from build123d import *

# Parameters (mm, degrees)
PAD_DEPTH     = 26.9875
SKETCH001_R   = 25
SKETCH001_R_2 = 15.925
PAD001_DEPTH  = 35
SKETCH002_R   = 25
SKETCH002_R_2 = 20
PAD002_DEPTH  = 381
SKETCH003_R   = 3.175
POCKET_DEPTH  = 12.7


with BuildPart() as part:
    # Sketch → Pad (new body, symmetric)
    with BuildSketch(Plane.YZ):
        Polygon((-25.4, -76.2), (-139.7, -76.2), (-139.7, 0), (0, 0), (0, -50.8), align=None)
    extrude(amount=PAD_DEPTH, both=True)

    # Sketch001 (on Face3 of Pad) → Pad001 (join)
    with BuildSketch(Plane(origin=(0, 0, 0), x_dir=(0, -1, 0), z_dir=(0, 0, 1))):
        with Locations((65, 0)):
            Circle(SKETCH001_R)
        with Locations((65, 0)):
            Circle(SKETCH001_R_2, mode=Mode.SUBTRACT)
    extrude(amount=PAD001_DEPTH)

    # Sketch002 → Pad002 (join)
    with BuildSketch(Plane.XZ):
        with Locations((0, -35.194401)):
            Circle(SKETCH002_R)
        with Locations((0, -35.194401)):
            Circle(SKETCH002_R_2, mode=Mode.SUBTRACT)
    extrude(amount=PAD002_DEPTH)

    # Sketch003 (on Face1 of Pad002) → Pocket (cut)
    with BuildSketch(Plane.YX.offset(76.2)):
        with Locations((-127, 0)):
            Circle(SKETCH003_R)
        with Locations((-95.25, 0)):
            Circle(SKETCH003_R)
    extrude(amount=-POCKET_DEPTH, mode=Mode.SUBTRACT)


solid = part.part
Verification items for the finished model (mm, model axes). A direction names the side the tool comes from. Coordinates: 2 decimals unless noted, no trailing zeros. Order: outer loops, then holes, each group sorted by start corner. A loop starts at its lowest first (then second) coordinate and runs counter-clockwise, first axis right, second up. Notation, with made-up numbers: M -33.75,8 L -7.75,8 A22 ccw -7.75,38 Z; hole C 72,35.25 d7. An arc over 180 degrees is marked long. Return JSON: item names as keys, results as strings.
1) Cross-section at D-D, the plane y = -150. Record the boundary of the cut face in (x, z), and give its area (3 significant figures).
Answer list:
{"outline": "C 0,-35.19 d50; hole C 0,-35.19 d40", "area": "707 mm2"}
2) Release check for a two-part mould opening along X. For faces 1 (the flat face through (0, -139.7, -64)), 2 (the cylindrical face through (-0.314, -4.159, -60.192)), 3 (the flat face through (0, -127, -63.5)) record: +X half, -X half, draft (parallel to the pull), parting line (faces both ways), or undercut.
Answer list:
{"face 1": "draft", "face 2": "parting line", "face 3": "undercut"}
3) Cross-section at B-B, the plane z = 9.5. Record the boundary of the cut face in (x, y) (3 decimals), and give its area (3 significant figures).
Answer list:
{"outline": "C 0,-65 d50; hole C 0,-65 d31.85", "area": "1,170 mm2"}
4) Cross-section at A-A, the plane y = -65. Record the boundary of the cut face in (x, z) (1 decimal).
Answer list:
{"outline": "M -27,-76.2 L 27,-76.2 L 27,0 L 25,0 L 25,35 L 15.9,35 L 15.9,0 L -15.9,0 L -15.9,35 L -25,35 L -25,0 L -27,0 Z"}
5) Access from +Z, -Z, +X, -X, +Y, -Y to the whole of each face (thin tool, end or side, straight path). Record for faces 4 (the cylindrical face through (-6.1, -79.71, 17.26)), 5 (the flat face through (0.4, -81.3, 35)), 6 (the cylindrical face through (-3.255, -258.661, -10.407)), 7 (the flat face through (0, -95, -63.5)).
Answer list:
{"face 4": "+Z", "face 5": "+Z, +X, -X, +Y, -Y", "face 6": "-Y", "face 7": "-Z"}
6) Cross-section at C-C, the plane x = -9. Record the boundary of the cut face in (y, z).
Answer list:
{"outline": "M -381,-58.52 L -139.7,-58.52 L -139.7,-76.2 L -25.4,-76.2 L -7.72,-58.52 L 0,-58.52 L 0,-53.05 L -2.25,-53.05 L 0,-50.8 L 0,0 L -41.68,0 L -41.68,35 L -51.86,35 L -51.86,0 L -78.14,0 L -78.14,35 L -88.32,35 L -88.32,0 L -139.7,0 L -139.7,-11.87 L -381,-11.87 L -381,-17.33 L -139.7,-17.33 L -139.7,-53.05 L -381,-53.05 Z"}
7) Thickness scan on L1, parallel to X at y = -95.25, z = -70 (1 decimal); L2, parallel to Y at x = -2.5, z = -65; L3, parallel to Y at x = -6, z = -37. Record the ranges inside material, lowest first. Write a range as [from, to].
Answer list:
{"L1": "[-27, -3.2], [3.2, 27]", "L2": "[-139.7, -128.96], [-125.04, -97.21], [-93.29, -14.2]", "L3": "[-139.7, 0]"}
8) Gauge pin test, flat ends, axial feed: pin 1 (7.5 mm diameter, centred on x = 0, y = -127, fed in from +Z); pin 2 (5 mm diameter, centred on y = -213, z = -22, fed in from +X); pin 3 (1.9 mm diameter, centred on x = 1, y = -128.5, fed in from -Z). Record the tip position at first contact, or that the pin passes through.
Answer list:
{"pin 1": "z = 0", "pin 2": "x = 22.6", "pin 3": "z = -63.5"}
